```python
from build123d import *

# Parameters (mm, degrees)
SKETCH1_R               = 1.75
BOSS_EXTRUDE1_DEPTH     = 4.1
CUT_EXTRUDE1_DEPTH      = 2
FILLET2_R               = 30
REDONDEO2_R             = 5
CORTAR_EXTRUIR1_DEPTH   = 3.5
SIMETR_A4_COPY_1_DEPTH  = 3.5
CROQUIS2_R              = 1.75
CORTAR_EXTRUIR2_DEPTH   = 2.5
CROQUIS3_R              = 1.75
SALIENTE_EXTRUIR1_DEPTH = 2.5


with BuildPart() as part:
    # Sketch1 → Boss-Extrude1 (new body)
    with BuildSketch(Plane(origin=(0, 0, 0), x_dir=(1, 0, 0), z_dir=(0, 1, 0))):
        Polygon((-27.516424079, 50), (27.516424079, 50), (38.33273811, 51.060660172), (51.060660172, 38.33273811), (50, 27.516424079), (50, -27.516424079), (51.060660172, -38.33273811), (38.33273811, -51.060660172), (27.516424079, -50), (-27.516424079, -50), (-38.33273811, -51.060660172), (-51.060660172, -38.33273811), (-50, -27.516424079), (-50, 27.516424079), (-51.060660172, 38.33273811), (-38.33273811, 51.060660172), align=None)
        with Locations(Location((-46.110912703, 37.625631329, 0), (0, 0, 270))):
            Circle(SKETCH1_R, mode=Mode.SUBTRACT)
        with Locations(Location((-37.625631329, 46.110912703, 0), (0, 0, 270))):
            Circle(SKETCH1_R, mode=Mode.SUBTRACT)
        with Locations(Location((-37.625631329, -46.110912703, 0), (0, 0, 270))):
            Circle(SKETCH1_R, mode=Mode.SUBTRACT)
        with Locations(Location((-46.110912703, -37.625631329, 0), (0, 0, 270))):
            Circle(SKETCH1_R, mode=Mode.SUBTRACT)
        with Locations(Location((46.110912703, -37.625631329, 0), (0, 0, 270))):
            Circle(SKETCH1_R, mode=Mode.SUBTRACT)
        with Locations(Location((37.625631329, -46.110912703, 0), (0, 0, 270))):
            Circle(SKETCH1_R, mode=Mode.SUBTRACT)
        with Locations(Location((46.110912703, 37.625631329, 0), (0, 0, 270))):
            Circle(SKETCH1_R, mode=Mode.SUBTRACT)
        with Locations(Location((37.625631329, 46.110912703, 0), (0, 0, 270))):
            Circle(SKETCH1_R, mode=Mode.SUBTRACT)
    extrude(amount=BOSS_EXTRUDE1_DEPTH)

    # Sketch2 → Cut-Extrude1 (cut)
    with BuildSketch(Plane(origin=(0, 4.1, 0), x_dir=(1, 0, 0), z_dir=(0, 1, 0))):
        Polygon((-40, -30), (-40, 30), (-30, 40), (30, 40), (40, 30), (40, -30), (30, -40), (-30, -40), align=None)
    extrude(amount=-CUT_EXTRUDE1_DEPTH, mode=Mode.SUBTRACT)

    # Fillet2
    # the kernel refuses this fillet: 30 mm, written as the material it adds along each edge
    with BuildSketch(Plane(origin=(27.516424079, 0, -50), x_dir=(-1, 0, 0), z_dir=(0, 1, 0)), Plane(origin=(50, 0, -27.516424079), x_dir=(0.09759304388656845, 0, -0.9952264052892459), z_dir=(0, 1, 0)), Plane(origin=(50, 0, 27.516424079), x_dir=(0, 0, -1), z_dir=(0, 1, 0)), Plane(origin=(27.516424079, 0, 50), x_dir=(0.9952264052892461, 0, 0.09759304388656681), z_dir=(0, 1, 0)), Plane(origin=(-27.516424079, 0, 50), x_dir=(1, 0, 0), z_dir=(0, 1, 0)), Plane(origin=(-50, 0, 27.516424079), x_dir=(-0.09759304388656528, 0, 0.9952264052892461), z_dir=(0, 1, 0)), Plane(origin=(-50, 0, -27.516424079), x_dir=(0, 0, 1), z_dir=(0, 1, 0))) as fillet2_piece_1:
        with BuildLine():
            CenterArc((FILLET2_R * 0.048913268002, -FILLET2_R), FILLET2_R, 90, 5.600584003)
            Line((-FILLET2_R * 0.0486797758846, -FILLET2_R * 0.00477359471075), (0, 0))
            Line((0, 0), (FILLET2_R * 0.048913268002, 0))
        make_face()
    extrude(amount=4.1)
    with BuildSketch(Plane(origin=(-27.516424079, 0, -50), x_dir=(1, 0, 0), z_dir=(0, 1, 0))) as fillet2_piece_2:
        with BuildLine():
            CenterArc((FILLET2_R * 0.048913268002, FILLET2_R), FILLET2_R, 264.399415997, 5.600584003)
            Line((-FILLET2_R * 0.0486797758846, FILLET2_R * 0.00477359471075), (0, 0))
            Line((0, 0), (FILLET2_R * 0.048913268002, 0))
        make_face()
    extrude(amount=4.1)

    # Redondeo2
    redondeo2_edges = [part.edges().sort_by_distance(p)[0] for p in [
        (38.33273811, 2.05, -51.060660172),
        (51.060660172, 2.05, -38.33273811),
        (51.060660172, 2.05, 38.33273811),
        (38.33273811, 2.05, 51.060660172),
        (-38.33273811, 2.05, 51.060660172),
        (-51.060660172, 2.05, 38.33273811),
        (-51.060660172, 2.05, -38.33273811),
        (-38.33273811, 2.05, -51.060660172),
    ]]
    fillet(redondeo2_edges, radius=REDONDEO2_R)

    # Croquis1 → Cortar-Extruir1 (cut)
    with BuildSketch(Plane(origin=(0, 4.1, 0), x_dir=(1, 0, 0), z_dir=(0, 1, 0))):
        Polygon((-18.354551733, -17.15), (-16.709103466, -20), (-18.354551733, -22.85), (-21.645448267, -22.85), (-23.290896534, -20), (-21.645448267, -17.15), align=None)
    cortar_extruir1 = extrude(amount=-CORTAR_EXTRUIR1_DEPTH, mode=Mode.SUBTRACT)

    # Simetría3: Cortar-Extruir1 across plane
    add(cortar_extruir1.mirror(Plane(origin=(0, 0, 0), x_dir=(0, 0, 1), z_dir=(1, 0, 0))), mode=Mode.SUBTRACT)

    # Simetría4: Cortar-Extruir1 across plane
    add(cortar_extruir1.mirror(Plane.XY), mode=Mode.SUBTRACT)

    # Simetría4 copy 1 sketch → Simetría4 copy 1 (cut)
    with BuildSketch(Plane(origin=(0, 4.1, 0), x_dir=(-1, 0, 0), z_dir=(0, 1, 0))):
        Polygon((-18.354551733, -17.15), (-16.709103466, -20), (-18.354551733, -22.85), (-21.645448267, -22.85), (-23.290896534, -20), (-21.645448267, -17.15), align=None)
    extrude(amount=-SIMETR_A4_COPY_1_DEPTH, mode=Mode.SUBTRACT)

    # Croquis2 → Cortar-Extruir2 (cut)
    with BuildSketch(Plane(origin=(0, 2.1, 0), x_dir=(1, 0, 0), z_dir=(0, 1, 0))):
        with Locations(Location((-20, -20, 0), (0, 0, 270))):
            Circle(CROQUIS2_R)
        with Locations(Location((-20, 20, 0), (0, 0, 270))):
            Circle(CROQUIS2_R)
        with Locations(Location((20, 20, 0), (0, 0, 270))):
            Circle(CROQUIS2_R)
        with Locations(Location((20, -20, 0), (0, 0, 270))):
            Circle(CROQUIS2_R)
    extrude(amount=-CORTAR_EXTRUIR2_DEPTH, mode=Mode.SUBTRACT)

    # Croquis3 → Saliente-Extruir1 (add)
    # profile 1 of 4: a face of its own
    with BuildSketch(Plane(origin=(0, 4.1, 0), x_dir=(1, 0, 0), z_dir=(0, 1, 0))):
        with BuildLine():
            Line((-49.389398906, 32.932931564), (-48.682292125, 32.225824783))
            ThreePointArc((-48.682292125, 32.225824783), (-46.560971781, 31.347145126), (-44.439651438, 32.225824783))
            Line((-44.439651438, 32.225824783), (-32.225824783, 44.439651438))
            ThreePointArc((-32.225824783, 44.439651438), (-31.347145126, 46.560971781), (-32.225824783, 48.682292125))
            Line((-32.225824783, 48.682292125), (-32.932931564, 49.389398906))
            ThreePointArc((-32.932931564, 49.389398906), (-36.46846547, 50.853865), (-40.003999376, 49.389398906))
            Line((-40.003999376, 49.389398906), (-49.389398906, 40.003999376))
            ThreePointArc((-49.389398906, 40.003999376), (-50.853865, 36.46846547), (-49.389398906, 32.932931564))
        make_face()
        with Locations(Location((-37.625631329, 46.110912703, 0), (0, 0, 270))):
            Circle(CROQUIS3_R, mode=Mode.SUBTRACT)
        with Locations(Location((-46.110912703, 37.625631329, 0), (0, 0, 270))):
            Circle(CROQUIS3_R, mode=Mode.SUBTRACT)
    # profile 2 of 4: a face of its own
    with BuildSketch(Plane(origin=(0, 4.1, 0), x_dir=(1, 0, 0), z_dir=(0, 1, 0))):
        with BuildLine():
            Line((-40.003999376, -49.389398906), (-49.389398906, -40.003999376))
            ThreePointArc((-49.389398906, -40.003999376), (-50.853865, -36.46846547), (-49.389398906, -32.932931564))
            Line((-49.389398906, -32.932931564), (-48.682292125, -32.225824783))
            ThreePointArc((-48.682292125, -32.225824783), (-46.560971781, -31.347145126), (-44.439651438, -32.225824783))
            Line((-44.439651438, -32.225824783), (-32.225824783, -44.439651438))
            ThreePointArc((-32.225824783, -44.439651438), (-31.347145126, -46.560971781), (-32.225824783, -48.682292125))
            Line((-32.225824783, -48.682292125), (-32.932931564, -49.389398906))
            ThreePointArc((-32.932931564, -49.389398906), (-36.46846547, -50.853865), (-40.003999376, -49.389398906))
        make_face()
        with Locations(Location((-46.110912703, -37.625631329, 0), (0, 0, 90))):
            Circle(CROQUIS3_R, mode=Mode.SUBTRACT)
        with Locations(Location((-37.625631329, -46.110912703, 0), (0, 0, 90))):
            Circle(CROQUIS3_R, mode=Mode.SUBTRACT)
    # profile 3 of 4: a face of its own
    with BuildSketch(Plane(origin=(0, 4.1, 0), x_dir=(1, 0, 0), z_dir=(0, 1, 0))):
        with BuildLine():
            Line((40.003999376, 49.389398906), (49.389398906, 40.003999376))
            ThreePointArc((49.389398906, 40.003999376), (50.853865, 36.46846547), (49.389398906, 32.932931564))
            Line((49.389398906, 32.932931564), (48.682292125, 32.225824783))
            ThreePointArc((48.682292125, 32.225824783), (46.560971781, 31.347145126), (44.439651438, 32.225824783))
            Line((44.439651438, 32.225824783), (32.225824783, 44.439651438))
            ThreePointArc((32.225824783, 44.439651438), (31.347145126, 46.560971781), (32.225824783, 48.682292125))
            Line((32.225824783, 48.682292125), (32.932931564, 49.389398906))
            ThreePointArc((32.932931564, 49.389398906), (36.46846547, 50.853865), (40.003999376, 49.389398906))
        make_face()
        with Locations(Location((46.110912703, 37.625631329, 0), (0, 0, 90))):
            Circle(CROQUIS3_R, mode=Mode.SUBTRACT)
        with Locations(Location((37.625631329, 46.110912703, 0), (0, 0, 90))):
            Circle(CROQUIS3_R, mode=Mode.SUBTRACT)
    # profile 4 of 4: a face of its own
    with BuildSketch(Plane(origin=(0, 4.1, 0), x_dir=(1, 0, 0), z_dir=(0, 1, 0))):
        with BuildLine():
            Line((49.389398906, -32.932931564), (48.682292125, -32.225824783))
            ThreePointArc((48.682292125, -32.225824783), (46.560971781, -31.347145126), (44.439651438, -32.225824783))
            Line((44.439651438, -32.225824783), (32.225824783, -44.439651438))
            ThreePointArc((32.225824783, -44.439651438), (31.347145126, -46.560971781), (32.225824783, -48.682292125))
            Line((32.225824783, -48.682292125), (32.932931564, -49.389398906))
            ThreePointArc((32.932931564, -49.389398906), (36.46846547, -50.853865), (40.003999376, -49.389398906))
            Line((40.003999376, -49.389398906), (49.389398906, -40.003999376))
            ThreePointArc((49.389398906, -40.003999376), (50.853865, -36.46846547), (49.389398906, -32.932931564))
        make_face()
        with Locations(Location((37.625631329, -46.110912703, 0), (0, 0, 270))):
            Circle(CROQUIS3_R, mode=Mode.SUBTRACT)
        with Locations(Location((46.110912703, -37.625631329, 0), (0, 0, 270))):
            Circle(CROQUIS3_R, mode=Mode.SUBTRACT)
    extrude(amount=SALIENTE_EXTRUIR1_DEPTH)


solid = part.part
```
Design review of the part built by this model. Coordinates are the model's own, in mm. A direction names the side the tool comes from. Give positions to 0.01 mm unless a question says otherwise; leave off trailing zeros. Write each loop counter-clockwise with the first axis right and the second up, starting at its lowest first coordinate (ties: lowest second). Pieces come first, ordered by that corner, then holes. Notation, with made-up numbers: (19, 40.25) -> (49, 40.25) arc R25 ccw to (49, 71.25) -> close; hole circle Ø7 at (49.25, 5). An arc over 180 degrees is marked (long way). Answer in a Markdown table with one row per item.
(1) Consider section C-C (x = 13.5). State the section outline as (y, z) points, then the cut area to 3 significant figures.
Results:
| item | result |
|---|---|
| outline | (0, -50) -> (4.1, -50) -> (4.1, -40) -> (2.1, -40) -> (2.1, 40) -> (4.1, 40) -> (4.1, 50) -> (0, 50) -> close |
| area | 250 mm2 |
(2) Consider section B-B (z = 5). State the section outline as (x, y) points, then the cut area to 3 significant figures.
Results:
| item | result |
|---|---|
| outline | (-50, 0) -> (50, 0) -> (50, 4.1) -> (40, 4.1) -> (40, 2.1) -> (-40, 2.1) -> (-40, 4.1) -> (-50, 4.1) -> close |
| area | 250 mm2 |
(3) For faces 5 (the flat face through (50.49, 2.02, -32.53)), 6 (the flat face through (38.418, 5.332, 38.247)), 7 (the cylindrical face through (-35.88, 3.25, 46.23)), 8 (the cylindrical face through (-27.535, 2.021, -50.037)), list the 3-axis set-ups (+Z, -Z, +X, -X, +Y, -Y) from which the entire face can be reached by the end or side of a thin tool; tool diameter is ignored.
Results:
| item | result |
|---|---|
| face 5 | +X, +Y, -Y |
| face 6 | +Y |
| face 7 | +Y, -Y |
| face 8 | -Z, +Y, -Y |
(4) Consider section A-A (x = -20). State the section outline as (y, z) points.
Results:
| item | result |
|---|---|
| outline | (0, -50) -> (4.1, -50) -> (4.1, -40) -> (2.1, -40) -> (2.1, -22.85) -> (0.6, -22.85) -> (0.6, -21.75) -> (0, -21.75) -> close; (0, -18.25) -> (0.6, -18.25) -> (0.6, -17.15) -> (2.1, -17.15) -> (2.1, 17.15) -> (0.6, 17.15) -> (0.6, 18.25) -> (0, 18.25) -> close; (0, 21.75) -> (0.6, 21.75) -> (0.6, 22.85) -> (2.1, 22.85) -> (2.1, 40) -> (4.1, 40) -> (4.1, 50) -> (0, 50) -> close |
(5) Mouldability with a two-part tool opening along Z and no side actions: class faces 1 (the flat face through (-32.43, 2.02, 50.48)), 2 (the flat face through (-32.53, 2.02, -50.49)), 3 (the cylindrical face through (47.857, 3.254, -37.51)), 4 (the cylindrical face through (45.046, 3.254, 36.237)) as +Z half, -Z half, draft (parallel to the pull), parting line (faces both ways), or undercut.
Results:
| item | result |
|---|---|
| face 1 | +Z half |
| face 2 | -Z half |
| face 3 | undercut |
| face 4 | undercut |
(6) To check wall thickness, follow probe 1 along X at (y, z) = (0.3, -20); probe 2 along Z at (x, y) = (-26, 3.5). State the ranges of each line that lie inside material, in increasing order.
Results:
| item | result |
|---|---|
| probe 1 | -50 to -21.75, -18.25 to 18.25, 21.75 to 50 |
| probe 2 | -50 to -40, 40 to 50 |
(7) Clearance check with flat-ended pins moving along their axes: pin 1 (1.6 mm diameter, centred on x = -19.5, y = 1.5, fed in from +Z); pin 2 (1.6 mm diameter, centred on x = -20, y = 1.5, fed in from -Z); pin 3 (3 mm diameter, centred on x = 20, z = 20, fed in from +Y); pin 4 (3 mm diameter, centred on x = 19, z = -20.5, fed in from +Y). State where each tip first meets the part, or that it passes through.
Results:
| item | result |
|---|---|
| pin 1 | z = 50 |
| pin 2 | z = -50 |
| pin 3 | through |
| pin 4 | y = 0.6 |
